Geometry check sheet. Reference: the model listing, model coordinates, mm. A direction names the side the tool comes from. Round coordinates to 2 decimals unless told otherwise and drop trailing zeros. Loops run counter-clockwise (first coordinate to the right, second up) from the corner with the lowest first, then second, coordinate; pieces in that order, holes last. Notation, with made-up numbers: (-10, 61) -> (27, 61) arc R25 ccw to (27, 96) -> close; hole circle Ø10 at (-6, -7.5). An arc over 180 degrees is marked (long way). Use one line per item in the form item = value.
from build123d import *

# Parameters (mm, degrees)
SCALE1_SCALE        = 0.222222222
SKETCH5_W           = 42.55
SKETCH5_H           = 39.12
BOSS_EXTRUDE1_DEPTH = 3


with BuildPart() as part:
    # Sketch2 → Loft1 section 0
    with BuildSketch(Plane.XY, mode=Mode.PRIVATE) as loft1_s0:
        with BuildLine():
            Line((0.798818744, 61.79823623), (-13.627719918, 19.2760512))
            Line((-13.627719918, 19.2760512), (-58.526766695, 19.856426989))
            Line((-58.526766695, 19.856426989), (-22.543811151, -7.004104425))
            Line((-22.543811151, -7.004104425), (-36.970349813, -49.526289455))
            Line((-36.970349813, -49.526289455), (-0.305121609, -23.604825795))
            Line((-0.305121609, -23.604825795), (35.677833934, -50.465357209))
            Line((35.677833934, -50.465357209), (22.355235626, -7.584480215))
            Line((22.355235626, -7.584480215), (59.020463829, 18.336983445))
            Line((59.020463829, 18.336983445), (14.121417053, 18.917359235))
            Line((14.121417053, 18.917359235), (0.798818744, 61.79823623))
        make_face()
    loft([loft1_s0.sketch, Vertex(0, 0, 20)])


with BuildPart() as part_1:
    # Scale1: scaled about (0, 0, 0)
    add(part.part.scale(SCALE1_SCALE))

    # Sketch5 → Boss-Extrude1 (add)
    with BuildSketch(Plane(origin=(0, 0, 0), x_dir=(-1, 0, 0), z_dir=(0, 0, -1))):
        Rectangle(SKETCH5_W, SKETCH5_H)
    extrude(amount=BOSS_EXTRUDE1_DEPTH)


solid = part_1.part
1. Tool access check on faces 5 (the flat face through (6.1, 0.956, 1.574)), 6 (the flat face through (-4.373, -4.359, 1.574)), 7 (the flat face through (-4, 5, 0)). Record the directions out of +Z, -Z, +X, -X, +Y, -Y that give a thin tool (end or side, any length) a straight path to the whole face; none if there is none.
Return value:
face_5 = +Z, +X
face_6 = +Z, -X
face_7 = +Z
2. Section check A-A (y = 12). Record the boundary of the cut face in (x, z) (3 decimals), then the cut area to 3 significant figures.
Return value:
outline = (-21.275, -3) -> (21.275, -3) -> (21.275, 0) -> (0.716, 0) -> (0.155, 0.561) -> (-0.41, 0) -> (-21.275, 0) -> close
area = 128 mm2
3. Section check C-C (x = -3.5). Record the boundary of the cut face in (y, z).
Return value:
outline = (-19.56, -3) -> (19.56, -3) -> (19.56, 0) -> (4.29, 0) -> (1.19, 3.25) -> (-1.09, 1.34) -> (-4.69, 2.55) -> (-7.67, 0) -> (-19.56, 0) -> close
4. Gauge pin test, flat ends, axial feed: pin 1 (12 mm diameter, centred on x = 13, y = -10, fed in from +Z); pin 2 (6 mm diameter, centred on x = 0, y = 6, fed in from +Z); pin 3 (6 mm diameter, centred on x = -4.5, y = -12.5, fed in from +Z). Record the tip position at first contact, or that the pin passes through.
Return value:
pin_1 = 0.52
pin_2 = 3.47
pin_3 = 0
5. Section check B-B (z = 0.5). Record the boundary of the cut face in (x, y).
Return value:
outline = (-11.54, 3.92) -> (-4.45, -1.38) -> (-7.29, -9.77) -> (-0.06, -4.66) -> (7.04, -9.95) -> (4.41, -1.5) -> (11.64, 3.62) -> (2.79, 3.73) -> (0.16, 12.19) -> (-2.69, 3.8) -> close
6. Mould release check, pull along X, two halves, no side actions. Record for faces 1 (the flat face through (4.427, -4.482, 1.41)), 2 (the flat face through (2.79, -5.51, 1.57)), 3 (the flat face through (0, 0, -3)), 4 (the flat face through (-21.275, 0, -1)): released by +X, released by -X, zero draft, split by the parting line, or undercut.
Return value:
face_1 = released by +X
face_2 = undercut
face_3 = zero draft
face_4 = released by -X
7. Section check D-D (x = 1.5). Record the boundary of the cut face in (y, z).
Return value:
outline = (-19.56, -3) -> (19.56, -3) -> (19.56, 0) -> (9.48, 0) -> (2.01, 2.32) -> (0.47, 3.94) -> (-0.51, 3.1) -> (-2.12, 3.6) -> (-6.42, 0) -> (-19.56, 0) -> close
8. Material ranges on line 1 along Z through (x, y) = (14, -7.5); line 2 along X through (y, z) = (-3, 0.25); line 3 along Z through (x, y) = (5.5, -5.5), recorded low to high.
Return value:
line_1 = -3 to 0
line_2 = -5.25 to 5.13
line_3 = -3 to 0.65
